Design review of the part built by this model. Coordinates are the model's own, in mm. Round coordinates to 2 decimals unless told otherwise and drop trailing zeros.
Autodesk Inventor part; units mm, degrees
ref_plane "YZ Plane" through (0, 0, 0) normal (1, 0, 0) x (0, 1, 0)
ref_plane "XZ Plane" through (0, 0, 0) normal (0, 1, 0) x (-1, 0, 0)
ref_plane "XY Plane" through (0, 0, 0) normal (0, 0, 1) x (1, 0, 0)
sketch "Sketch1" plane through (0, 0, 0) normal (0, 1, 0) x (-1, 0, 0)
  line L0 (0, 0) -> (38.1, 0)
  line L1 (38.1, 0) -> (38.1, -88.9)
  line L2 (38.1, -88.9) -> (0, -88.9)
  line L3 (0, -88.9) -> (0, 0)
  dimension "d0" = 38.1
  dimension "d1" = 88.9
extrude "Extrusion1" add sketch "Sketch1" along normal blind 2400.3
sketch "Sketch4" plane through (0, 0, 0) normal (0, -1, 0) x (1, 0, 0)
  line L0 (-38.1, -88.9) -> (-38.1, 0)
  line L1 (0, 0) -> (-38.1, 0)
  line L2 (-38.1, 0) -> (-38.1, -44.45)
  line L3 (-38.1, -44.45) -> (0, -44.45)
  line L4 (0, -44.45) -> (0, 0)
  line L5 (0, 0) -> (0, -88.9)
  line L6 (-19.05, -44.45) -> (0, -44.45)
  line L7 (0, -44.45) -> (0, -22.225)
  line L8 (0, -22.225) -> (-19.05, -22.225)
  line L9 (-19.05, -22.225) -> (-19.05, -44.45)
  circle A0 centre (-19.05, -22.225) radius 2.3812
  circle A1 centre (-19.05, -66.675) radius 2.3812
  dimension "d12" = 4.7625
extrude "Extrusion4" cut sketch "Sketch4" against normal blind 38.1 contours A0 L8 L9 | L9 L8 A0 | A1
sketch "Sketch5" plane through (0, 0, 0) normal (1, 0, 0) x (0, 0, -1)
  line L0 (88.9, 0) -> (88.9, 2400.3)
  line L1 (0, 0) -> (0, 2400.3)
  line L2 (88.9, 2400.3) -> (0, 2400.3)
  line L3 (0, 2400.3) -> (0, 2362.2)
  line L4 (0, 2362.2) -> (88.9, 2362.2)
  line L5 (88.9, 2362.2) -> (88.9, 2400.3)
  line L6 (0, 2362.2) -> (44.45, 2362.2)
  line L7 (44.45, 2362.2) -> (44.45, 2381.25)
  line L8 (44.45, 2381.25) -> (0, 2381.25)
  line L9 (0, 2381.25) -> (0, 2362.2)
  line L10 (44.45, 2381.25) -> (22.225, 2381.25)
  line L11 (22.225, 2381.25) -> (22.225, 2362.2)
  line L12 (22.225, 2362.2) -> (44.45, 2362.2)
  line L13 (44.45, 2362.2) -> (44.45, 2381.25)
  circle A0 centre (22.225, 2381.25) radius 2.3812
  circle A1 centre (66.675, 2381.25) radius 2.3812
  dimension "d15" = 38.1
  dimension "d16" = 4.7625
extrude "Extrusion5" cut sketch "Sketch5" against normal up to surface (38.1 mm away) contours A0 L8 L11 | L11 L8 A0 | L8 A0 | A1
properties part number "wallLeftLong" material "Wood (Birch)"
1) Clearance check with flat-ended pins moving along their axes: P1, Ø6, axis at y = 2381.25, z = -22.225, coming from the -X side; P2, Ø1.4, axis at x = -19, z = -66, coming from the -Y side. State where each tip first meets the part, or that it passes through.
Results:
P1: stops at x = -38.1
P2: stops at y = 38.1
2) To check wall thickness, follow line 1 along Z through (x, y) = (-27.5, 2381.25); line 2 along Y through (x, z) = (-31, -66.5). State the ranges of each line that lie inside material, in increasing order.
Results:
line 1: z = -88.9 to -69.06, -64.29 to -24.61, -19.84 to 0
line 2: y = 0 to 2378.88, 2383.62 to 2400.3
3) The part is to be moulded in two halves that separate along Z. For faces 1 (the face through (-19, 1183, -88.9)), 2 (the face through (-19, 1183, 0)), 3 (the face through (-19, 0, -44)), say which applies: released by +Z, released by -Z, zero draft, split by the parting line, or undercut.
Results:
face 1: released by -Z
face 2: released by +Z
face 3: zero draft
